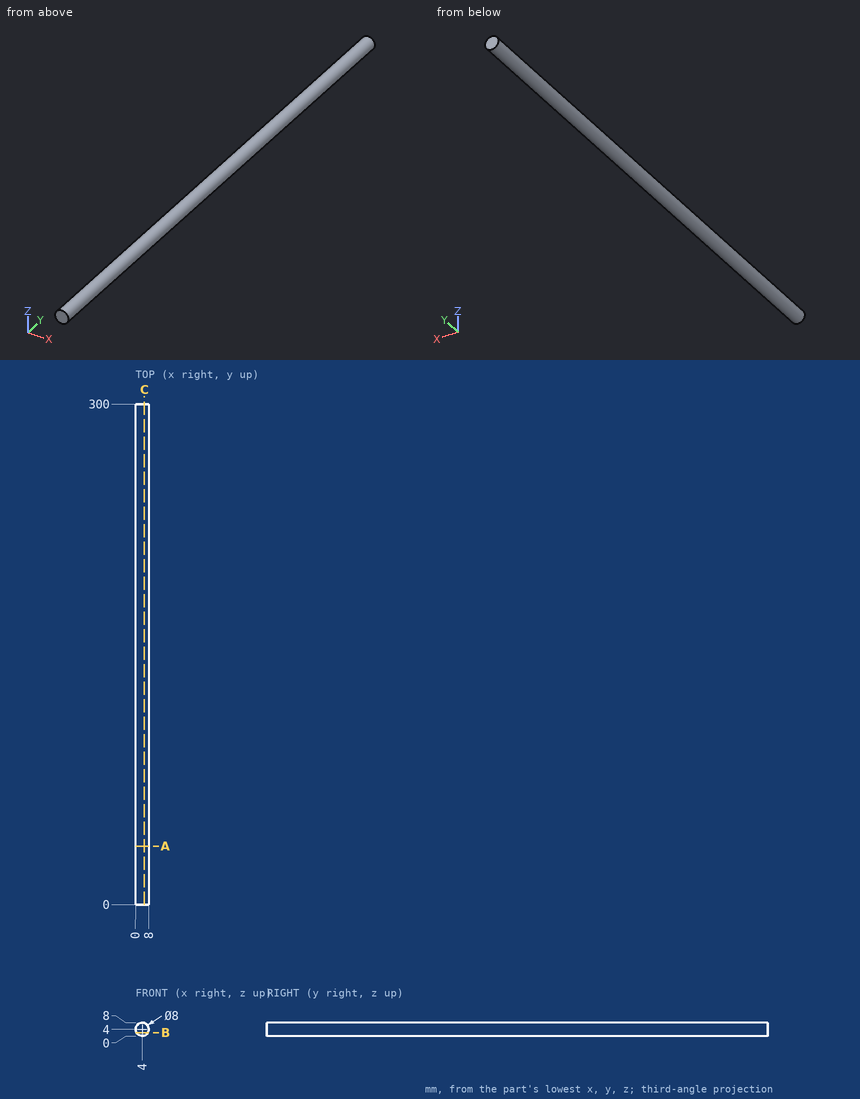
Input: dimensioned drawing with shaded views. Units: mm. Origin: part minimum x, y, z. Round coordinates to 2 decimals unless told otherwise and drop trailing zeros. Loops run counter-clockwise (first coordinate to the right, second up) from the corner with the lowest first, then second, coordinate; pieces in that order, holes last. Notation, with made-up numbers: (-27.5, 42.5) -> (20.5, 42.5) arc R20 ccw to (20.5, 58.5) -> close; hole circle Ø10 at (38.25, 77.25). An arc over 180 degrees is marked (long way). Answer as a JSON object with one key per item and string values. Group by question number.
Q1. Ray query, line 1 (X direction, y = 33, z = 3.5); line 2 (Z direction, x = 7.25, y = 66); line 3 (X direction, y = 31.5, z = 6.25). Return the intervals inside material, ascending. Write a range as from..to.
Q2. Section query C-C (x = 5.25). Output: boundary loops of the cut face in (y, z), plus the area to 3 significant figures.
Q3. Section query A-A (y = 35). Output: boundary loops of the cut face in (x, z).
Q4. Contact query for a flat-ended pin moving along its axis: P1, Ø1.5, axis at y = 31.5, z = 6, coming from the -X side. Output: stop coordinate, or through.
Q5. Section query B-B (z = 2). Output: boundary loops of the cut face in (x, y), plus the area to 3 significant figures.
Completed:
{
 "1": {"line 1": "0.03..7.97", "line 2": "1.67..6.33", "line 3": "0.69..7.31"},
 "2": {"outline": "(0, 0.2) -> (300, 0.2) -> (300, 7.8) -> (0, 7.8) -> close", "area": "2,280 mm²"},
 "3": {"outline": "circle Ø8 at (4, 4)"},
 "4": {"P1": "x = 0.2"},
 "5": {"outline": "(0.54, 0) -> (7.46, 0) -> (7.46, 300) -> (0.54, 300) -> close", "area": "2,080 mm²"}
}
